Autodesk Inventor part; units mm, degrees
ref_plane "YZ Plane" through (0, 0, 0) normal (1, 0, 0) x (0, 1, 0)
ref_plane "XZ Plane" through (0, 0, 0) normal (0, 1, 0) x (-1, 0, 0)
ref_plane "XY Plane" through (0, 0, 0) normal (0, 0, 1) x (1, 0, 0)
sketch "スケッチ1" plane through (0, 0, 0) normal (0, 0, 1) x (1, 0, 0)
  line L0 (0, 44.5) -> (30, 44.5)
  line L1 (0, 0) -> (30, 0)
  line L2 (0, 0) -> (0, 44.5)
  line L3 (30, 0) -> (30, 44.5)
  line L4 (7.5, 0) -> (7.5, 5)
  line L5 (7.5, 5) -> (22.5, 5)
  line L6 (15, 0) -> (15, 44.5) construction
  line L7 (22.5, 0) -> (22.5, 5)
  line L8 (5, 36.5) -> (25, 36.5)
  line L9 (25, 36.5) -> (25, 7.5)
  line L10 (25, 7.5) -> (5, 7.5)
  line L11 (5, 36.5) -> (5, 7.5)
  point P0 (22.5, 0)
  dimension "d2" = 30
  dimension "d38" = 44.5
  dimension "d61" = 15
  dimension "d62" = 5
  dimension "d66" = 5
  dimension "d67" = 8
  dimension "d68" = 2.5
extrude "押し出し1" add sketch "スケッチ1" along normal blind 5 contours L0 L3 L1 L7 L5 L4 L2
sketch "スケッチ4" plane through (30, 0, 0) normal (1, 0, 0) x (0, 0, -1)
  line L0 (0, 44.5) -> (-5, 44.5)
  line L1 (-2.5, 44.5) -> (-2.5, 0) construction
  line L2 (0, 0) -> (-5, 0)
  point P0 (0, 0)
  point P1 (-2.5, 39.5)
  point P2 (-2.5, 2.5)
  point P3 (-2.5, 7.5)
  point P4 (-2.5, 12.5)
  dimension "d22" = 5
  dimension "d40" = 2.5
  dimension "d41" = 5
  dimension "d42" = 5
  dimension "d60" = 27
hole "穴1" at (30, 39.5, 2.5) direction (-1, 0, 0) diameter 3.1 depth 3
sketch "スケッチ5" plane through (0, 0, 0) normal (-1, 0, 0) x (0, 0, 1)
  circle A0 centre (2.5, 39.5) radius 1.55
  line L0 (0, 0) -> (5, 0)
  line L1 (2.5, 0) -> (2.5, 44.5) construction
  line L2 (0, 44.5) -> (5, 44.5)
  point P0 (2.5, 2.5)
  point P1 (2.5, 7.5)
  point P2 (2.5, 12.5)
  point P3 (4.05, 32)
  point P4 (0.95, 32)
  dimension "d50" = 2.5
  dimension "d51" = 5
  dimension "d52" = 5
hole "穴2" at (0, 39.5, 2.5) direction (1, 0, 0) diameter 3.1 depth 3
hole "穴5" at (30, 2.5, 2.5) at (30, 12.5, 2.5) at (30, 7.5, 2.5) direction (-1, 0, 0) diameter 2.9 depth 3
hole "穴6" at (0, 2.5, 2.5) at (0, 7.5, 2.5) at (0, 12.5, 2.5) direction (1, 0, 0) diameter 2.9 depth 3
extrude "押し出し2" add sketch "スケッチ1" along normal blind 2.5 contours L4 L5 L7 L1
fillet "フィレット3" radius 2 8 edges at (7.5, 5, 3.75) (7.5, 0, 3.75) (22.5, 5, 3.75) (22.5, 0, 3.75) (5, 36.5, 2.5) (25, 36.5, 2.5) (5, 7.5, 2.5) (25, 7.5, 2.5)
extrude "押し出し3" add sketch "スケッチ1" along normal blind 1 contours L8 L9 L10 L11
properties part number "Cockpit_vertical_frame_07" material "アセタール樹脂、黒"
Work out the finished part from the listing and answer in its coordinate system (mm). A direction names the side the tool comes from. Give positions to 0.01 mm unless a question says otherwise; leave off trailing zeros. Loops run counter-clockwise (first coordinate to the right, second up) from the corner with the lowest first, then second, coordinate; pieces in that order, holes last. Notation, with made-up numbers: (-18, -0.5) -> (13, -0.5) arc R27 cw to (13, 29.5) -> close; hole circle Ø10 at (36.25, 52.5). An arc over 180 degrees is marked (long way). Use a Markdown table: item, result. Add a question column.
1. Section B-B on y = 39.5 is taken. Determine the outline of the cut face in (x, z), and give its area (3 significant figures).
2. Find the intervals of material crossed by probe 1 along Y at (x, z) = (1.4, 2.5); probe 2 along Z at (x, y) = (1.9, 12.5); probe 3 along X at (y, z) = (33.5, 1.6), in increasing order.
3. Section A-A on x = 28.25 is taken. Determine the outline of the cut face in (y, z).
4. Section C-C on x = 13 is taken. Determine the outline of the cut face in (y, z), and give its area (3 significant figures).
5. Determine the mould class of faces 5 (the flat face through (27, 2, 3)), 6 (the cylindrical face through (21.93, 4.4, 3.77)), 7 (the flat face through (22.5, 2.5, 3.7)) for opening direction Y: released by +Y, released by -Y, zero draft, split by the parting line, or undercut.
6. For faces 1 (the cylindrical face through (24.43, 35.9, 3.03)), 2 (the cylindrical face through (8.1, 4.43, 3.77)), 3 (the cylindrical face through (28.479, 41.013, 2.836)), 4 (the flat face through (3, 7, 2)), determine the directions among +Z, -Z, +X, -X, +Y, -Y from which every point of the face is accessible in a straight line to the end or side of a thin tool.
7. Flat-ended cylindrical pins translate along their axes: pin 1 Ø2.5 at (y, z) = (2.5, 2.5) entering from -X; pin 2 Ø1.2 at (x, z) = (14, 4) entering from -Y; pin 3 Ø10 at (x, y) = (11.5, 27.5) entering from +Z. Find the tip coordinate at first contact, or state that the pin passes through.
8. Section D-D on y = 2.5 is taken. Determine the outline of the cut face in (x, z), and give its area (3 significant figures).
Results below:
| question | item | result |
|---|---|---|
| 1 | outline | (0, 0) -> (30, 0) -> (30, 0.95) -> (27, 0.95) -> (27, 4.05) -> (30, 4.05) -> (30, 5) -> (0, 5) -> (0, 4.05) -> (3, 4.05) -> (3, 0.95) -> (0, 0.95) -> close |
| 1 | area | 131 mm^2 |
| 2 | probe 1 | y = 0 to 1.05, 3.95 to 6.05, 8.95 to 11.05, 13.95 to 37.95, 41.05 to 44.5 |
| 2 | probe 2 | z = 0 to 1.05, 3.95 to 5 |
| 2 | probe 3 | x = 0 to 5, 25 to 30 |
| 3 | outline | (0, 0) -> (44.5, 0) -> (44.5, 5) -> (0, 5) -> close; hole circle Ø2.9 at (2.5, 2.5); hole circle Ø2.9 at (7.5, 2.5); hole circle Ø2.9 at (12.5, 2.5); hole circle Ø3.1 at (39.5, 2.5) |
| 4 | outline | (0, 0) -> (44.5, 0) -> (44.5, 5) -> (36.5, 5) -> (36.5, 1) -> (7.5, 1) -> (7.5, 5) -> (5, 5) -> (5, 2.5) -> (0, 2.5) -> close |
| 4 | area | 94.0 mm^2 |
| 5 | face 5 | undercut |
| 5 | face 6 | released by -Y |
| 5 | face 7 | zero draft |
| 6 | face 1 | +Z |
| 6 | face 2 | +Z, -Y |
| 6 | face 3 | +X |
| 6 | face 4 | -X |
| 7 | pin 1 | stops at x = 3 |
| 7 | pin 2 | stops at y = 5 |
| 7 | pin 3 | stops at z = 1 |
| 8 | outline | (0, 0) -> (30, 0) -> (30, 1.05) -> (27, 1.05) -> (27, 3.95) -> (30, 3.95) -> (30, 5) -> (22.5, 5) -> (22.5, 2.5) -> (7.5, 2.5) -> (7.5, 5) -> (0, 5) -> (0, 3.95) -> (3, 3.95) -> (3, 1.05) -> (0, 1.05) -> close |
| 8 | area | 95.1 mm^2 |
